The listing builds one solid part. Answer for the finished solid, in the listing's coordinates (mm). A direction names the side the tool comes from. Coordinates: 2 decimals unless noted, no trailing zeros. Write each loop counter-clockwise with the first axis right and the second up, starting at its lowest first coordinate (ties: lowest second). Pieces come first, ordered by that corner, then holes.
(1) Straight lines are drawn through the part: line 1 (X direction, y = 13.25, z = 0); line 2 (Y direction, x = 15, z = 1); line 3 (Z direction, x = 3, y = 4.75). For each, find the intervals that lie inside material, in ascending order.
(2) The part is cut by section B-B on y = 11.5. Determine the outline of the cut face in (x, z), plus the area to 3 significant figures.
(3) The part is cut by section A-A on x = 0. Determine the outline of the cut face in (y, z).
(4) For a pull along Z with two mould halves and no side action, classify faces 3 (the cylindrical face through (-10.648, 8.874, -13.887)), 4 (the cylindrical face through (-13.765, 14.056, -0.228)), 5 (the flat face through (0, 0, 0)) as +Z half, -Z half, draft (parallel to the pull), parting line (faces both ways), or undercut.
(5) The part is cut by section D-D on y = 2.75. Determine the outline of the cut face in (x, z).
(6) The part is cut by section C-C on z = 0. Determine the outline of the cut face in (x, y).
(7) Which of the six approach directions +Z, -Z, +X, -X, +Y, -Y give full straight-line access (tool end or side, diameter ignored) to faces 1 (the flat face through (16, 10, 0)), 2 (the flat face through (-4, 18, 0))?
(8) Given P1, Ø6, axis at x = -6.5, y = 8, coming from the +Z side; P2, Ø1.5, axis at y = 10.5, z = 11.5, coming from the +X side; P3, Ø1.8, axis at x = 0.5, z = 1.5, coming from the +Y side, each flat-ended and moving along its own axis, determine where each tip first touches the part or whether it passes through.
from build123d import *

# Parameters (mm, degrees)
SKETCH_1_R          = 17.5
EXTRUDE_1_DEPTH     = 18
SKETCH_2_R          = 3
CUT_EXTRUDE_1_DEPTH = 12
SKETCH_3_R          = 1.75
CUT_EXTRUDE_2_DEPTH = 8


with BuildPart() as part:
    # 草图1 → 凸台-拉伸1 (new body)
    with BuildSketch(Plane(origin=(0, 0, 0), x_dir=(1, 0, 0), z_dir=(0, 1, 0))):
        with Locations(Location((0, 0, 0), (0, 0, 270))):
            Circle(SKETCH_1_R)
    extrude(amount=EXTRUDE_1_DEPTH)

    # 草图2 → 切除-拉伸1 (cut)
    with BuildSketch(Plane(origin=(0, 18, 0), x_dir=(1, 0, 0), z_dir=(0, 1, 0))):
        with Locations(Location((0, 0, 0), (0, 0, 270))):
            Circle(SKETCH_2_R)
    extrude(amount=-CUT_EXTRUDE_1_DEPTH, mode=Mode.SUBTRACT)

    # 草图3 → 切除-拉伸2 (cut)
    with BuildSketch(Plane(origin=(0, 18, 0), x_dir=(1, 0, 0), z_dir=(0, 1, 0))):
        with Locations(Location((15.5, 0, 0), (0, 0, 270))):
            Circle(SKETCH_3_R)
        with Locations(Location((-15.5, 0, 0), (0, 0, 270))):
            Circle(SKETCH_3_R)
    extrude(amount=-CUT_EXTRUDE_2_DEPTH, mode=Mode.SUBTRACT)


solid = part.part
Model answer:
1. line 1: x = -17.5 to -17.25, -13.75 to -3, 3 to 13.75, 17.25 to 17.5
1. line 2: y = 0 to 10
1. line 3: z = -17.24 to 17.24
2. outline: circle Ø35 at (0, 0); hole circle Ø3.5 at (-15.5, 0); hole circle Ø6 at (0, 0); hole circle Ø3.5 at (15.5, 0)
2. area: 915 mm2
3. outline: (0, -17.5) - (18, -17.5) - (18, -3) - (6, -3) - (6, 3) - (18, 3) - (18, 17.5) - (0, 17.5) - close
4. face 3: parting line
4. face 4: undercut
4. face 5: draft
5. outline: circle Ø35 at (0, 0)
6. outline: (-17.5, 0) - (17.5, 0) - (17.5, 18) - (17.25, 18) - (17.25, 10) - (13.75, 10) - (13.75, 18) - (3, 18) - (3, 6) - (-3, 6) - (-3, 18) - (-13.75, 18) - (-13.75, 10) - (-17.25, 10) - (-17.25, 18) - (-17.5, 18) - close
7. face 1: +Y
7. face 2: +Z, -Z, +X, -X, +Y
8. P1: stops at z = 17.15
8. P2: stops at x = 13.81
8. P3: stops at y = 6
